```python
from build123d import *

# Parameters (mm, degrees)
SKETCH1_W             = 16
SKETCH1_H             = 96
SKETCH1_R             = 3
BOSS_EXTRUDE1_DEPTH   = 17
BOSS_EXTRUDE1_2_DEPTH = 17
SKETCH2_W             = 91
SKETCH2_H             = 96
BOSS_EXTRUDE2_DEPTH   = 83
SKETCH3_R             = 41
BOSS_EXTRUDE3_DEPTH   = 36
BOSS_EXTRUDE4_REACH   = 98
SKETCH4_R             = 6.5
SKETCH5_R             = 36
BOSS_EXTRUDE5_DEPTH   = 8.5
SKETCH6_R             = 25
CUT_EXTRUDE1_DEPTH    = 1
DOME1_FACE_RADIUS     = 25
DOME1_HEIGHT          = 16
SKETCH7_R             = 6.5
SKETCH7_R_2           = 3.5
BOSS_EXTRUDE6_DEPTH   = 9


with BuildPart() as part:
    # Sketch1 → Boss-Extrude1 (new body)
    with BuildSketch(Plane(origin=(0, 0, 0), x_dir=(1, 0, 0), z_dir=(0, 1, 0))):
        with Locations((-31.5, 0)):
            Rectangle(SKETCH1_W, SKETCH1_H)
        with Locations((-32, 40.5)):
            Circle(SKETCH1_R, mode=Mode.SUBTRACT)
        with Locations((-32, -40.5)):
            Circle(SKETCH1_R, mode=Mode.SUBTRACT)
    extrude(amount=BOSS_EXTRUDE1_DEPTH)



with BuildPart() as body_2:
    # Sketch1 → Boss-Extrude1 2 (new body)
    with BuildSketch(Plane(origin=(0, 0, 0), x_dir=(1, 0, 0), z_dir=(0, 1, 0))):
        with Locations((31.5, 0)):
            Rectangle(SKETCH1_W, SKETCH1_H)
        with Locations((32, 40.5)):
            Circle(SKETCH1_R, mode=Mode.SUBTRACT)
        with Locations((32, -40.5)):
            Circle(SKETCH1_R, mode=Mode.SUBTRACT)
    extrude(amount=BOSS_EXTRUDE1_2_DEPTH)


with BuildPart() as part_1:
    add(part.part)

    add(body_2.part)  # Boss-Extrude2 merges body 2
    # Sketch2 → Boss-Extrude2 (add)
    with BuildSketch(Plane(origin=(0, 17, 0), x_dir=(1, 0, 0), z_dir=(0, 1, 0))):
        with Locations((6, 0)):
            Rectangle(SKETCH2_W, SKETCH2_H)
    extrude(amount=BOSS_EXTRUDE2_DEPTH)

    # Sketch3 → Boss-Extrude3 (add)
    with BuildSketch(Plane.ZY.offset(39.5)):
        with Locations((0, 50)):
            Circle(SKETCH3_R)
    extrude(amount=BOSS_EXTRUDE3_DEPTH)

    # Sketch4 → Boss-Extrude4 (add, up to next)
    with BuildSketch(Plane.XY.offset(48), mode=Mode.PRIVATE) as boss_extrude4_sk1:
        with Locations((-59.5, 28)):
            Circle(SKETCH4_R)
    boss_extrude4_tool1 = extrude(boss_extrude4_sk1.sketch, amount=-BOSS_EXTRUDE4_REACH, mode=Mode.PRIVATE) - part_1.part
    add(boss_extrude4_tool1.solids().sort_by_distance((-59.5, 28, 48))[0])

    # Sketch5 → Boss-Extrude5 (add)
    with BuildSketch(Plane(origin=(51.5, 0, 0), x_dir=(0, 0, -1), z_dir=(1, 0, 0))):
        with Locations((0, 58.5)):
            Circle(SKETCH5_R)
    extrude(amount=BOSS_EXTRUDE5_DEPTH)

    # Sketch6 → Cut-Extrude1 (cut)
    with BuildSketch(Plane(origin=(60, 0, 0), x_dir=(0, 0, -1), z_dir=(1, 0, 0))):
        with Locations((0, 58.5)):
            Circle(SKETCH6_R)
    extrude(amount=-CUT_EXTRUDE1_DEPTH, mode=Mode.SUBTRACT)

    # Dome1: a dome of height H over a round flat face of radius A is a cap of a sphere of radius (A * A + H * H) / (2 * H)
    dome1_r = (DOME1_FACE_RADIUS * DOME1_FACE_RADIUS + DOME1_HEIGHT * DOME1_HEIGHT) / (2 * DOME1_HEIGHT)
    dome1_base = Plane((59, 58.5, 0), z_dir=(1, 0, 0))
    with Locations(dome1_base.offset(DOME1_HEIGHT - dome1_r)):
        dome1_ball = Sphere(dome1_r, mode=Mode.PRIVATE)
    add(split(dome1_ball, bisect_by=dome1_base, keep=Keep.TOP, mode=Mode.PRIVATE))

    # Sketch7 → Boss-Extrude6 (add, symmetric)
    with BuildSketch(Plane(origin=(75, 0, 0), x_dir=(0, 0, -1), z_dir=(1, 0, 0))):
        with Locations((0, 58.5)):
            Circle(SKETCH7_R)
        with Locations((0, 58.5)):
            Circle(SKETCH7_R_2, mode=Mode.SUBTRACT)
    extrude(amount=BOSS_EXTRUDE6_DEPTH, both=True)


solid = part_1.part
```
Build history of the part. All positions in model axes, mm. A direction names the side the tool comes from. Give positions to 0.01 mm unless a question says otherwise; leave off trailing zeros. Loops run counter-clockwise (first coordinate to the right, second up) from the corner with the lowest first, then second, coordinate; pieces in that order, holes last. Notation, with made-up numbers: (40, 67) - (93, 67) arc R18 ccw to (93, 89) - close; hole circle Ø4 at (35.25, -31.75). An arc over 180 degrees is marked (long way). Use a Markdown table: item, result.
(1) Wall check: line 1 along Z through (x, y) = (32.5, 12.5); line 2 along X through (y, z) = (12.75, 40.5); line 3 along Y through (x, z) = (78, 0). Give the ranges that are in metal, low to high.
Taken from the geometry:
| item | result |
|---|---|
| line 1 | -48 to -43.46, -37.54 to 37.54, 43.46 to 48 |
| line 2 | -39.5 to -35, -29 to -23.5, 23.5 to 29, 35 to 39.5 |
| line 3 | 52 to 55, 62 to 65 |
(2) Which spindle directions (+Z, -Z, +X, -X, +Y, -Y) get a long thin tool onto all of the face, cutting with end or side? Do faces 5 (the face through (55.69, 94.194, 4.686)), 6 (the face through (23.5, 8, 1)), 7 (the face through (-60.909, 21.655, 40.925)). Say none if no direction does.
Taken from the geometry:
| item | result |
|---|---|
| face 5 | +X |
| face 6 | +Z, -Z, -Y |
| face 7 | +Z |
(3) Band-saw the part on C-C (z = 10.5). Give the cut face in (x, y), and give its area (3 significant figures).
Taken from the geometry:
| item | result |
|---|---|
| outline | (-75.5, 10.37) - (-39.5, 10.37) - (-39.5, 0) - (-23.5, 0) - (-23.5, 17) - (23.5, 17) - (23.5, 0) - (39.5, 0) - (39.5, 17) - (51.5, 17) - (51.5, 24.07) - (60, 24.07) - (60, 35.81) - (59, 35.81) arc R25.45 ccw to (59, 81.19) - (60, 81.19) - (60, 92.93) - (51.5, 92.93) - (51.5, 100) - (-39.5, 100) - (-39.5, 89.63) - (-75.5, 89.63) - close |
| area | 11,900 mm2 |
(4) Drop flat-ended pins along their axis: pin 1 Ø5 at (x, z) = (33.5, -39.5) entering from -Y; pin 2 Ø3.5 at (x, z) = (46.5, -2.5) entering from -Y; pin 3 Ø10 at (x, z) = (-46, -10) entering from -Y; pin 4 Ø1.5 at (y, z) = (17, 4.5) entering from +X. Give the stop position or say it passes through.
Taken from the geometry:
| item | result |
|---|---|
| pin 1 | y = 0 |
| pin 2 | y = 17 |
| pin 3 | y = 9.31 |
| pin 4 | x = 51.5 |
(5) Band-saw the part on A-A (x = 32). Give the cut face in (y, z).
Taken from the geometry:
| item | result |
|---|---|
| outline | (0, -48) - (100, -48) - (100, 48) - (0, 48) - (0, 43.5) - (17, 43.5) - (17, 37.5) - (0, 37.5) - (0, -37.5) - (17, -37.5) - (17, -43.5) - (0, -43.5) - close |
(6) Band-saw the part on B-B (y = 58.5). Give the cut face in (x, z), and give its area (3 significant figures).
Taken from the geometry:
| item | result |
|---|---|
| outline | (-75.5, -40.11) - (-39.5, -40.11) - (-39.5, -48) - (51.5, -48) - (51.5, -36) - (60, -36) - (60, -25) - (59, -25) arc R27.53 ccw to (74.22, -6.5) - (84, -6.5) - (84, -3.5) - (74.78, -3.5) arc R27.53 ccw to (74.78, 3.5) - (84, 3.5) - (84, 6.5) - (74.22, 6.5) arc R27.53 ccw to (59, 25) - (60, 25) - (60, 36) - (51.5, 36) - (51.5, 48) - (-39.5, 48) - (-39.5, 40.11) - (-75.5, 40.11) - close |
| area | 12,800 mm2 |
(7) Band-saw the part on D-D (y = 80). Give the cut face in (x, z), and give its area (3 significant figures).
Taken from the geometry:
| item | result |
|---|---|
| outline | (-75.5, -27.95) - (-39.5, -27.95) - (-39.5, -48) - (51.5, -48) - (51.5, -28.87) - (60, -28.87) - (60, -12.76) - (59, -12.76) arc R17.2 ccw to (59, 12.76) - (60, 12.76) - (60, 28.87) - (51.5, 28.87) - (51.5, 48) - (-39.5, 48) - (-39.5, 27.95) - (-75.5, 27.95) - close |
| area | 11,300 mm2 |
(8) Pull direction Z, two halves, no side cores. Call faces 1 (the face through (29.79, 8.38, 38.47)), 2 (the face through (0, 17, -1)), 3 (the face through (5, 49, -48)), 4 (the face through (29.79, 8.38, -42.53)): +Z half, -Z half, draft (parallel to the pull), parting line (faces both ways), or undercut.
Taken from the geometry:
| item | result |
|---|---|
| face 1 | undercut |
| face 2 | draft |
| face 3 | -Z half |
| face 4 | undercut |
